Autodesk Fusion 360 part; units mm, degrees
sketch "Sketch1" plane through (0, 0, 0) normal (0, 1, 0) x (1, 0, 0)
  line L0 (0, 0) -> (0, -20) construction
  line L1 (0, -20) -> (30, -20)
  line L2 (30, -20) -> (30, 0)
  line L3 (30, 0) -> (20, 0)
  line L4 (20, 0) -> (20, 20)
  line L5 (20, 20) -> (0, 20)
  line L6 (-20, 0) -> (-20, 20)
  line L7 (-30, 0) -> (-20, 0)
  line L8 (-30, -20) -> (-30, 0)
  line L9 (-20, 20) -> (0, 20)
  line L10 (0, -20) -> (-30, -20)
  dimension "d1" = 20
  dimension "d2" = 30
extrude "Extrude1" add sketch "Sketch1" along normal blind 15
sketch "Sketch2" plane through (0, 0, 0) normal (0, -1, 0) x (1, 0, 0)
  line L0 (30, 0) -> (30, 20)
  line L1 (30, 20) -> (-30, 20)
  line L2 (-30, 20) -> (-30, 0)
  line L3 (-30, 0) -> (-20, 0)
  line L4 (-20, 0) -> (-20, -20)
  line L5 (-20, -20) -> (20, -20)
  line L6 (20, -20) -> (20, 0)
  line L7 (20, 0) -> (30, 0)
  line L8 (30, 20) -> (38, 20)
  line L9 (38, 20) -> (38, 0)
  line L10 (38, 0) -> (30, 0)
  line L11 (30, 0) -> (30, 20)
  line L12 (-30, 20) -> (-38, 20)
  line L13 (-38, 20) -> (-38, 0)
  line L14 (-38, 0) -> (-30, 0)
  line L15 (-30, 0) -> (-30, 20)
  dimension "d5" = 8
  dimension "d6" = 8
  dimension "d7" = 20
extrude "Extrude2" add sketch "Sketch2" along normal blind 3
sketch "Sketch3" plane through (0, -3, 0) normal (0, -1, 0) x (1, 0, 0)
  line L0 (38, 20) -> (-38, 20)
  line L1 (-38, 20) -> (-38, 0)
  line L2 (-38, 0) -> (-20, 0)
  line L3 (-20, 0) -> (-20, -20)
  line L4 (-20, -20) -> (20, -20)
  line L5 (20, -20) -> (20, 0)
  line L6 (20, 0) -> (38, 0)
  line L7 (38, 0) -> (38, 20)
  line L8 (-30, 20) -> (-30, 0)
  line L9 (0, 20) -> (-30, 20)
  line L10 (30, 20) -> (30, 0)
  line L11 (0, 20) -> (30, 20)
  line L12 (30, 0) -> (20, 0)
  line L13 (20, 0) -> (20, -20)
  line L14 (20, -20) -> (0, -20)
  line L15 (-20, -20) -> (0, -20)
  line L16 (-20, 0) -> (-20, -20)
  line L17 (-30, 0) -> (-20, 0)
extrude "Extrude3" add sketch "Sketch3" along normal blind 5 contours L0 L2 L3 L4 L5 L6 L8 L9 L10 L11 L12 L13 L14 L15 L16 L17
fillet "Fillet1" radius 2.5 2 edges at (38, -3, 10) (-38, -3, 10)
sketch "Sketch4" plane through (0, -8, 0) normal (0, -1, 0) x (1, 0, 0)
  line L0 (30, 20) -> (-30, 20)
  line L1 (-30, 20) -> (-30, 0)
  line L2 (-30, 0) -> (-20, 0)
  line L3 (-20, 0) -> (-20, -20)
  line L4 (-20, -20) -> (20, -20)
  line L5 (20, -20) -> (20, 0)
  line L6 (20, 0) -> (30, 0)
  line L7 (30, 0) -> (30, 20)
  line L8 (-20, -10) -> (20, -10) construction
  line L9 (20, 0) -> (20, -20)
  line L10 (-5.5, 20) -> (0, 20)
  line L11 (0, 20) -> (0, 13.9)
  line L12 (0, 13.9) -> (-5.5, 13.9)
  line L13 (-5.5, 13.9) -> (-5.5, 20)
  line L14 (0, 13.9) -> (5.5, 13.9)
  line L15 (5.5, 13.9) -> (5.5, 20)
  line L16 (5.5, 20) -> (0, 20)
  line L17 (14.8575, 20) -> (-15.1425, 20)
  line L18 (-15.1425, 20) -> (-15.1425, 10.5)
  line L19 (-15.1425, 10.5) -> (14.8575, 10.5)
  line L20 (14.8575, 10.5) -> (14.8575, 20)
  line L21 (14.8575, 20) -> (-15.1425, 10.5) construction
  line L22 (-15.1425, 20) -> (14.8575, 10.5) construction
  line L23 (9.65, 0) -> (-9.65, 0)
  line L24 (-9.65, 0) -> (-9.65, 10.5)
  line L25 (-9.65, 10.5) -> (9.65, 10.5)
  line L26 (9.65, 10.5) -> (9.65, 0)
  line L27 (9.65, 0) -> (-9.65, 10.5) construction
  line L28 (-9.65, 0) -> (9.65, 10.5) construction
  line L29 (5.5, 13.9) -> (14.8575, 13.9)
  line L30 (-15.1425, 13.9) -> (-5.5, 13.9)
  line L31 (-5.5, 13.9) -> (-5.5, 10.5)
  line L32 (5.5, 13.9) -> (5.5, 10.5)
  point P0 (-10, -10)
  point P1 (10, -10)
  point P2 (-0.1425, 15.25)
  point P3 (0, 5.25)
  dimension "d14" = 10
  dimension "d15" = 10
  dimension "d19" = 5.5
  dimension "d20" = 6.1
  dimension "d21" = 24.5
  dimension "d37" = 30
  dimension "d38" = 9.5
  dimension "d39" = 19.3
  dimension "d40" = 10.5
hole "Hole1" at (10, -8, -10) at (-10, -8, -10) direction (0, 1, 0) diameter 5.5 end through all
extrude "Extrude4" cut sketch "Sketch4" against normal through all contours L0 L11 L14 L15 L16 L17 | L0 L10 L11 L12 L13 L17 | L12 L14 L19 L25 L31 L32 | L19 L23 L24 L25 L26
sketch "Sketch5" plane through (0, 15, 0) normal (0, 1, 0) x (-1, 0, 0)
  line L0 (-5.5, 20) -> (-30, 20)
  line L1 (-30, 20) -> (-30, 0)
  line L2 (-30, 0) -> (-20, 0)
  line L3 (-20, 0) -> (-20, -20)
  line L4 (-20, -20) -> (20, -20)
  line L5 (20, -20) -> (20, 0)
  line L6 (20, 0) -> (30, 0)
  line L7 (30, 0) -> (30, 20)
  line L8 (30, 20) -> (5.5, 20)
  circle A0 centre (-10, -10) radius 2.75
  circle A1 centre (10, -10) radius 2.75
  line L9 (0, 13.9) -> (0, -20) construction
  line L10 (-20, -10) -> (20, -10) construction
  line L11 (-16.55, -15.425) -> (-18.15, -15.425)
  line L12 (-18.15, -15.425) -> (-18.15, -4.575)
  line L13 (-18.15, -4.575) -> (-16.55, -4.575)
  line L14 (-16.55, -4.575) -> (-16.55, -15.425)
  line L15 (-16.55, -15.425) -> (-18.15, -4.575) construction
  line L16 (-18.15, -15.425) -> (-16.55, -4.575) construction
  line L17 (-13.95, -12.825) -> (-16.55, -12.825)
  line L18 (-16.55, -12.825) -> (-16.55, -7.175)
  line L19 (-16.55, -7.175) -> (-13.95, -7.175)
  line L20 (-13.95, -7.175) -> (-13.95, -12.825)
  line L21 (-13.95, -12.825) -> (-16.55, -7.175) construction
  line L22 (-16.55, -12.825) -> (-13.95, -7.175) construction
  line L23 (-16.55, -4.575) -> (-13.95, -7.175)
  line L24 (-13.95, -12.825) -> (-16.55, -15.425)
  line L25 (18.15, -4.575) -> (16.55, -4.575)
  line L26 (16.55, -4.575) -> (13.95, -7.175)
  line L27 (13.95, -7.175) -> (13.95, -12.825)
  line L28 (13.95, -12.825) -> (16.55, -15.425)
  line L29 (16.55, -15.425) -> (18.15, -15.425)
  line L30 (18.15, -15.425) -> (18.15, -4.575)
  line L31 (-30, 10) -> (30, 10) construction
  line L32 (-26.55, 4.575) -> (-28.15, 4.575)
  line L33 (-28.15, 4.575) -> (-28.15, 15.425)
  line L34 (-28.15, 15.425) -> (-26.55, 15.425)
  line L35 (-26.55, 15.425) -> (-26.55, 4.575)
  line L36 (-26.55, 4.575) -> (-28.15, 15.425) construction
  line L37 (-28.15, 4.575) -> (-26.55, 15.425) construction
  line L38 (-23.95, 7.175) -> (-26.55, 7.175)
  line L39 (-26.55, 7.175) -> (-26.55, 12.825)
  line L40 (-26.55, 12.825) -> (-23.95, 12.825)
  line L41 (-23.95, 12.825) -> (-23.95, 7.175)
  line L42 (-23.95, 7.175) -> (-26.55, 12.825) construction
  line L43 (-26.55, 7.175) -> (-23.95, 12.825) construction
  line L44 (-23.95, 12.825) -> (-26.55, 15.425)
  line L45 (-23.95, 7.175) -> (-26.55, 4.575)
  line L46 (23.95, 7.175) -> (26.55, 4.575)
  line L47 (23.95, 12.825) -> (23.95, 7.175)
  line L48 (23.95, 12.825) -> (26.55, 15.425)
  line L49 (28.15, 15.425) -> (26.55, 15.425)
  line L50 (28.15, 4.575) -> (28.15, 15.425)
  line L51 (26.55, 4.575) -> (28.15, 4.575)
  line L52 (5.5, 10.5) -> (9.65, 10.5)
  line L53 (9.65, 10.5) -> (9.65, 0)
  line L54 (9.65, 0) -> (-9.65, 0)
  line L55 (-9.65, 0) -> (-9.65, 10.5)
  line L56 (-9.65, 10.5) -> (-5.5, 10.5)
  line L57 (-5.5, 10.5) -> (-5.5, 20)
  line L58 (5.5, 20) -> (5.5, 10.5)
  point P0 (-17.35, -10)
  point P1 (-15.25, -10)
  point P2 (-27.35, 10)
  point P3 (-25.25, 10)
  dimension "d24" = 1.6
  dimension "d25" = 10.85
  dimension "d26" = 1.85
  dimension "d28" = 5.65
  dimension "d31" = 45
  dimension "d32" = 1.6
  dimension "d33" = 10.85
  dimension "d34" = 5.65
  dimension "d35" = 45
  dimension "d36" = 1.85
extrude "Extrude5" add sketch "Sketch5" along normal blind 5 contours L11 L12 L13 L14 L18 | L14 L17 L24 | L14 L17 L18 L19 L20 | L14 L19 L23 | L25 L26 L27 L28 L29 L30 | L32 L33 L34 L35 L39 | L35 L38 L45 | L35 L38 L39 L40 L41 | L35 L40 L44 | L46 L47 L48 L49 L50 L51
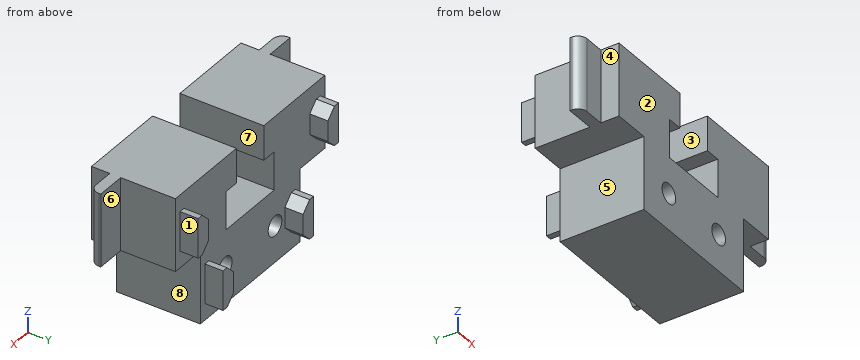
Read the model definition and answer for the solid it produces. Units are mm, in the model's axes. Face numbers are marked on the shaded views. A direction names the side the tool comes from. Round coordinates to 2 decimals unless told otherwise and drop trailing zeros. Write each loop counter-clockwise with the first axis right and the second up, starting at its lowest first coordinate (ties: lowest second). Pieces come first, ordered by that corner, then holes. Notation, with made-up numbers: (81.5, -40) -> (86.5, -40) arc R12 ccw to (86.5, -25) -> close; hole circle Ø8 at (14.5, -4.5). An arc over 180 degrees is marked (long way). Answer in a Markdown table with one row per item. Add a question column.
1) Find section C-C, the plane z = -10. Determine the outline of the cut face in (x, y).
2) Find section B-B, the plane y = 11.25. Determine the outline of the cut face in (x, z).
3) Find section A-A, the plane z = 3. Determine the outline of the cut face in (x, y), and give its area (3 significant figures).
4) Find section D-D, the plane z = 12. Determine the outline of the cut face in (x, y), and give its area (3 significant figures).
5) Which of the six approach directions +Z, -Z, +X, -X, +Y, -Y give full straight-line access (tool end or side, diameter ignored) to the marked faces 5, 6, 7 and 8?
6) Determine the mould class of the marked faces 1, 2, 3 and 4 for opening direction X: pulls with the +X half, pulls with the -X half, needs draft (parallel to the pull), parting line crosses it, or undercut.
7) Consider line 1 (X direction, y = 3.5, z = -10); line 2 (Z direction, x = -10, y = 5.75); line 3 (Z direction, x = 7, y = 12.75). Determine where each line is inside the solid, lowest interval first.
8) Given P1, Ø14.5, axis at x = 28, y = 0.5, coming from the -Z side; P2, Ø12, axis at x = 0.5, z = -13.5, coming from the +Y side; P3, Ø6, axis at y = 11.5, z = -2, coming from the +X side, each flat-ended and moving along its own axis, determine where each tip first touches the part or whether it passes through.
Findings below:
| question | item | result |
|---|---|---|
| 1 | outline | (-20, -8) -> (-12.75, -8) -> (-12.75, 15) -> (-13.95, 15) -> (-13.95, 20) -> (-18.15, 20) -> (-18.15, 15) -> (-20, 15) -> close; (-7.25, -8) -> (7.25, -8) -> (7.25, 15) -> (-7.25, 15) -> close; (12.75, -8) -> (20, -8) -> (20, 15) -> (18.15, 15) -> (18.15, 20) -> (13.95, 20) -> (13.95, 15) -> (12.75, 15) -> close |
| 2 | outline | (-30, 0) -> (-20, 0) -> (-20, -20) -> (20, -20) -> (20, 0) -> (30, 0) -> (30, 20) -> (5.5, 20) -> (5.5, 10.5) -> (9.65, 10.5) -> (9.65, 0) -> (-9.65, 0) -> (-9.65, 10.5) -> (-5.5, 10.5) -> (-5.5, 20) -> (-30, 20) -> close; hole circle Ø5.5 at (-10, -10); hole circle Ø5.5 at (10, -10) |
| 3 | outline | (-38, -0.5) arc R2.5 ccw to (-35.5, -3) -> (-30, -3) -> (-30, -8) -> (-9.65, -8) -> (-9.65, 15) -> (-30, 15) -> (-30, 0) -> (-38, 0) -> close; (9.65, -8) -> (30, -8) -> (30, -3) -> (35.5, -3) arc R2.5 ccw to (38, -0.5) -> (38, 0) -> (30, 0) -> (30, 15) -> (9.65, 15) -> close |
| 3 | area | 981 mm² |
| 4 | outline | (-38, -0.5) arc R2.5 ccw to (-35.5, -3) -> (-30, -3) -> (-30, -8) -> (-5.5, -8) -> (-5.5, 15) -> (-23.95, 15) -> (-23.95, 20) -> (-28.15, 20) -> (-28.15, 15) -> (-30, 15) -> (-30, 0) -> (-38, 0) -> close; (5.5, -8) -> (30, -8) -> (30, -3) -> (35.5, -3) arc R2.5 ccw to (38, -0.5) -> (38, 0) -> (30, 0) -> (30, 15) -> (28.15, 15) -> (28.15, 20) -> (23.95, 20) -> (23.95, 15) -> (5.5, 15) -> close |
| 4 | area | 1,210 mm² |
| 5 | face 5 | -Z, -X, +Y, -Y |
| 5 | face 6 | +Z, -Z, +X, +Y |
| 5 | face 7 | +Z, +Y, -Y |
| 5 | face 8 | -Z, +X, +Y, -Y |
| 6 | face 1 | pulls with the +X half |
| 6 | face 2 | needs draft |
| 6 | face 3 | undercut |
| 6 | face 4 | pulls with the -X half |
| 7 | line 1 | -20 to -12.75, -7.25 to 7.25, 12.75 to 20 |
| 7 | line 2 | -20 to -12.75, -7.25 to 20 |
| 7 | line 3 | -20 to 0, 10.5 to 20 |
| 8 | P1 | z = 0 |
| 8 | P2 | y = 15 |
| 8 | P3 | x = 30 |
